For this review, take the finished solid that the model builds, in its own axes (mm). Face numbers are marked on the shaded views. Round coordinates to 2 decimals unless told otherwise and drop trailing zeros. Order: outer loops, then holes, each group sorted by start corner. A loop starts at its lowest first (then second) coordinate and runs counter-clockwise, first axis right, second up. Notation, with made-up numbers: (8, 83) - (35, 83) arc R30 ccw to (35, 108) - close; hole circle Ø1 at (54, 15.25). An arc over 180 degrees is marked (long way). Write each question's results on one line, items separated by ' | '. Start each with the question number.
(1) Take a section at A-A, the plane y = -29. Give the boundary of the cut face in (x, z), plus the area to 3 significant figures.
(2) Take a section at C-C, the plane y = -7.5. Give the boundary of the cut face in (x, z).
(3) For L1, parallel to Y at x = 146, z = 10.25; L2, parallel to Y at x = 156.5, z = 12.55; L3, parallel to Y at x = 128, z = 2.5, list the stretches that pass through material, from the lowest coordinate up. Write a range as from..to.
(4) Take a section at B-B, the plane x = 118. Give the boundary of the cut face in (y, z), plus the area to 3 significant figures.
(5) Insertion check: pin 1 Ø1.2 at (y, z) = (29, 1.5) entering from -X; pin 2 Ø13.5 at (x, y) = (-15.5, -15.5) entering from +Z; pin 3 Ø2.5 at (y, z) = (1, 10.5) entering from +X; pin 4 Ø3 at (x, y) = (156.5, 29) entering from +Z. Each pin has a flat end and moves straight along its axis. Give the tip position at first contact, or say it passes through.
(6) Take a section at D-D, the plane x = -5. Give the boundary of the cut face in (y, z).
(7) Draft analysis for pull direction Z (two halves, no side actions). For the marked faces 1, 2, 3 and 4, state which applies: pulls with the +Z half, pulls with the -Z half, needs draft (parallel to the pull), parting line crosses it, or undercut.
```python
from build123d import *

# Parameters (mm, degrees)
CROQUIS1_W                        = 103
CROQUIS1_H                        = 103
CROQUIS1_R                        = 2.5
SALIENTE_EXTRUIR1_DEPTH           = 15
REDONDEO2_R                       = 51.5
CROQUIS2_W                        = 15
CROQUIS2_H                        = 103
SALIENTE_EXTRUIR2_DEPTH           = 120
CROQUIS3_R                        = 4.25
CORTAR_EXTRUIR1_DEPTH             = 8
SALIENTE_EXTRUIR3_START           = -223
SALIENTE_EXTRUIR3_DEPTH           = 223
CORTAR_EXTRUIR2_DEPTH             = 181.53669987
CORTAR_EXTRUIR2_DEPTH_BACK        = 181.53669987
REDONDEO3_START                   = -23.965772234
REDONDEO3_DEPTH                   = 195.465772234
REDONDEO3_START_2                 = -45.024993159
REDONDEO3_2_DEPTH                 = 21.059220925
REDONDEO3_START_3                 = 15
REDONDEO3_3_DEPTH                 = 9
REDONDEO4_R                       = 10
CORTAR_EXTRUIR3_REACH             = 182.537
CROQUIS6_R                        = 4.25
CORTAR_EXTRUIR3_DIRECTION_2_DEPTH = 181.536699978
CORTAR_EXTRUIR4_DEPTH             = 231.022281636
CORTAR_EXTRUIR4_DEPTH_BACK        = 40
CROQUIS7_W                        = 5
CROQUIS7_H                        = 80
CROQUIS10_R                       = 4.25
CORTAR_EXTRUIR5_DEPTH             = 10
CROQUIS11_R                       = 2.5
CORTAR_EXTRUIR6_DEPTH             = 180.536904387
CROQUIS12_W                       = 16
CROQUIS12_H                       = 24
CROQUIS12_W_2                     = 12
CROQUIS12_H_2                     = 20
SALIENTE_EXTRUIR4_DEPTH           = 171.5
CORTAR_EXTRUIR7_DEPTH             = 4
CROQUIS14_W                       = 242.583484446
CROQUIS14_H                       = 103.867159029
CORTAR_EXTRUIR8_DEPTH             = 8


with BuildPart() as part:
    # Croquis1 → Saliente-Extruir1 (new body)
    with BuildSketch(Plane.XY):
        Rectangle(CROQUIS1_W, CROQUIS1_H)
        with Locations((15.5, 15.5)):
            Circle(CROQUIS1_R, mode=Mode.SUBTRACT)
        with Locations((-15.5, 15.5)):
            Circle(CROQUIS1_R, mode=Mode.SUBTRACT)
        with Locations((-15.5, -15.5)):
            Circle(CROQUIS1_R, mode=Mode.SUBTRACT)
        with Locations((15.5, -15.5)):
            Circle(CROQUIS1_R, mode=Mode.SUBTRACT)
    extrude(amount=SALIENTE_EXTRUIR1_DEPTH)

    # Redondeo2
    redondeo2_edges = [part.edges().sort_by_distance(p)[0] for p in [
        (-51.5, -51.5, 7.5),
        (-51.5, 51.5, 7.5),
    ]]
    fillet(redondeo2_edges, radius=REDONDEO2_R - 0.0001)  # a hair under: the kernel refuses the full size

    # Croquis2 → Saliente-Extruir2 (add)
    with BuildSketch(Plane(origin=(51.5, 0, 0), x_dir=(0, 0, -1), z_dir=(1, 0, 0))):
        with Locations((-7.5, 0)):
            Rectangle(CROQUIS2_W, CROQUIS2_H)
    extrude(amount=SALIENTE_EXTRUIR2_DEPTH)

    # Croquis3 → Cortar-Extruir1 (cut)
    with BuildSketch(Plane.XY.offset(15)):
        with Locations((-15.5, 15.5)):
            Circle(CROQUIS3_R)
        with Locations((15.5, 15.5)):
            Circle(CROQUIS3_R)
        with Locations((15.5, -15.5)):
            Circle(CROQUIS3_R)
        with Locations((-15.5, -15.5)):
            Circle(CROQUIS3_R)
    extrude(amount=-CORTAR_EXTRUIR1_DEPTH, mode=Mode.SUBTRACT)

    # Croquis4 → Saliente-Extruir3 (add)
    with BuildSketch(Plane(origin=(171.5, 0, 0), x_dir=(0, 0, -1), z_dir=(1, 0, 0)).offset(SALIENTE_EXTRUIR3_START)):
        Polygon((-15, -19), (-15, -25), (-23, -25), (-23, 25), (-15, 25), (-15, 19), (-19, 19), (-19, -19), align=None)
    extrude(amount=SALIENTE_EXTRUIR3_DEPTH)

    # Croquis5 → Cortar-Extruir2 (cut, two sides: drawn at the far end of the back side and taken through both)
    with BuildSketch(Plane(origin=(0, 0, 0), x_dir=(-1, 0, 0), z_dir=(0, 0, -1)).offset(-CORTAR_EXTRUIR2_DEPTH_BACK)):
        with BuildLine():
            Line((40.930864284, 31.255629077), (61.422564692, 30.315306135))
            Line((61.422564692, 30.315306135), (63.075048064, -35.056936027))
            Line((63.075048064, -35.056936027), (38.432028807, -34.281615507))
            ThreePointArc((38.432028807, -34.281615507), (48.122237498, -18.343943366), (51.5, 0))
            ThreePointArc((51.5, 0), (48.786214808, 16.497128377), (40.930864284, 31.255629077))
        make_face()
    extrude(amount=CORTAR_EXTRUIR2_DEPTH + CORTAR_EXTRUIR2_DEPTH_BACK, mode=Mode.SUBTRACT)

    # Redondeo3: read off the stored shape, not the designer's step
    # Redondeo3 outline → Redondeo3 (add)
    with BuildSketch(Plane.YZ.offset(REDONDEO3_START)):
        with BuildLine():
            Line((-25, 15), (-25, 23))
            ThreePointArc((-25, 23), (-28.473403651, 17.254033308), (-34.797958971, 15))
            Line((-34.797958971, 15), (-25, 15))
        make_face()
        with BuildLine():
            ThreePointArc((34.797958971, 15), (28.473403651, 17.254033308), (25, 23))
            Line((25, 23), (25, 15))
            Line((25, 15), (34.797958971, 15))
        make_face()
    extrude(amount=REDONDEO3_DEPTH)

    # Redondeo3 2 outline → Redondeo3 2 (add)
    with BuildSketch(Plane.YZ.offset(REDONDEO3_START_2)):
        with BuildLine():
            ThreePointArc((34.797958971, 15), (28.473403651, 17.254033308), (25, 23))
            Line((25, 23), (25, 15))
            Line((25, 15), (34.797958971, 15))
        make_face()
        with BuildLine():
            Line((-25, 15), (-25, 23))
            ThreePointArc((-25, 23), (-28.473403651, 17.254033308), (-34.797958971, 15))
            Line((-34.797958971, 15), (-25, 15))
        make_face()
    extrude(amount=REDONDEO3_2_DEPTH)

    # Redondeo3 3 outline → Redondeo3 3 (cut)
    with BuildSketch(Plane.XY.offset(REDONDEO3_START_3)):
        with BuildLine():
            Line((-45.024993159, -36), (-36.827299657, -36))
            ThreePointArc((-36.827299657, -36), (-41.294060795, -30.774186311), (-45.024993083, -24.999999958))
            Line((-45.024993083, -24.999999958), (-45.024993159, -36))
        make_face()
        with BuildLine():
            Line((-45.024993159, 36), (-45.024993083, 24.999999958))
            ThreePointArc((-45.024993083, 24.999999958), (-41.294060795, 30.774186311), (-36.827299657, 36))
            Line((-36.827299657, 36), (-45.024993159, 36))
        make_face()
    extrude(amount=REDONDEO3_3_DEPTH, mode=Mode.SUBTRACT)

    # Redondeo4
    redondeo4_edges = [part.edges().sort_by_distance(p)[0] for p in [
        (63.237503445, -25, 23),
        (63.237503445, 25, 23),
    ]]
    fillet(redondeo4_edges, radius=REDONDEO4_R)

    # Croquis6 → Cortar-Extruir3 (cut, up to next)
    with BuildSketch(Plane.XY.offset(23), mode=Mode.PRIVATE) as cortar_extruir3_sk1:
        with Locations((15.5, 15.5)):
            Circle(CROQUIS6_R)
    cortar_extruir3_tool1 = extrude(cortar_extruir3_sk1.sketch, amount=-CORTAR_EXTRUIR3_REACH, mode=Mode.PRIVATE) & part.part
    # Croquis6 → Cortar-Extruir3 (cut, up to next)
    with BuildSketch(Plane.XY.offset(23), mode=Mode.PRIVATE) as cortar_extruir3_sk2:
        with Locations((-15.5, 15.5)):
            Circle(CROQUIS6_R)
    cortar_extruir3_tool2 = extrude(cortar_extruir3_sk2.sketch, amount=-CORTAR_EXTRUIR3_REACH, mode=Mode.PRIVATE) & part.part
    # Croquis6 → Cortar-Extruir3 (cut, up to next)
    with BuildSketch(Plane.XY.offset(23), mode=Mode.PRIVATE) as cortar_extruir3_sk3:
        with Locations((15.5, -15.5)):
            Circle(CROQUIS6_R)
    cortar_extruir3_tool3 = extrude(cortar_extruir3_sk3.sketch, amount=-CORTAR_EXTRUIR3_REACH, mode=Mode.PRIVATE) & part.part
    # Croquis6 → Cortar-Extruir3 (cut, up to next)
    with BuildSketch(Plane.XY.offset(23), mode=Mode.PRIVATE) as cortar_extruir3_sk4:
        with Locations((-15.5, -15.5)):
            Circle(CROQUIS6_R)
    cortar_extruir3_tool4 = extrude(cortar_extruir3_sk4.sketch, amount=-CORTAR_EXTRUIR3_REACH, mode=Mode.PRIVATE) & part.part
    add(cortar_extruir3_tool1.solids().sort_by_distance((15.5, 15.5, 23))[0], mode=Mode.SUBTRACT)
    add(cortar_extruir3_tool2.solids().sort_by_distance((-15.5, 15.5, 23))[0], mode=Mode.SUBTRACT)
    add(cortar_extruir3_tool3.solids().sort_by_distance((15.5, -15.5, 23))[0], mode=Mode.SUBTRACT)
    add(cortar_extruir3_tool4.solids().sort_by_distance((-15.5, -15.5, 23))[0], mode=Mode.SUBTRACT)

    # Croquis6 → Cortar-Extruir3 direction 2 (cut)
    with BuildSketch(Plane.XY.offset(23)):
        with Locations((15.5, 15.5)):
            Circle(CROQUIS6_R)
        with Locations((-15.5, 15.5)):
            Circle(CROQUIS6_R)
        with Locations((15.5, -15.5)):
            Circle(CROQUIS6_R)
        with Locations((-15.5, -15.5)):
            Circle(CROQUIS6_R)
    extrude(amount=CORTAR_EXTRUIR3_DIRECTION_2_DEPTH, mode=Mode.SUBTRACT)

    # Croquis7 → Cortar-Extruir4 (cut, two sides: drawn at the far end of the back side and taken through both)
    with BuildSketch(Plane(origin=(171.5, 0, 0), x_dir=(0, 0, -1), z_dir=(1, 0, 0)).offset(-CORTAR_EXTRUIR4_DEPTH_BACK)):
        with Locations((-9.5, 0)):
            Rectangle(CROQUIS7_W, CROQUIS7_H)
    extrude(amount=CORTAR_EXTRUIR4_DEPTH + CORTAR_EXTRUIR4_DEPTH_BACK, mode=Mode.SUBTRACT)

    # Croquis10 → Cortar-Extruir5 (cut)
    with BuildSketch(Plane.XY.offset(23)):
        with Locations((156.5, 29)):
            Circle(CROQUIS10_R)
        with Locations(Location((156.5, -29, 0), (0, 0, 31.206732466))):
            Circle(CROQUIS10_R)
    extrude(amount=-CORTAR_EXTRUIR5_DEPTH, mode=Mode.SUBTRACT)

    # Croquis11 → Cortar-Extruir6 (cut, through all)
    with BuildSketch(Plane.XY.offset(13)):
        with Locations((156.5, 29)):
            Circle(CROQUIS11_R)
        with Locations((156.5, -29)):
            Circle(CROQUIS11_R)
    extrude(amount=-CORTAR_EXTRUIR6_DEPTH, mode=Mode.SUBTRACT)

    # Croquis12 → Saliente-Extruir4 (add)
    with BuildSketch(Plane(origin=(171.5, 0, 0), x_dir=(0, 0, -1), z_dir=(1, 0, 0))):
        with Locations((-8, -63.5)):
            Rectangle(CROQUIS12_W, CROQUIS12_H)
        with Locations((-8, -63.5)):
            Rectangle(CROQUIS12_W_2, CROQUIS12_H_2, mode=Mode.SUBTRACT)
    extrude(amount=-SALIENTE_EXTRUIR4_DEPTH)

    # Croquis13 → Cortar-Extruir7 (cut)
    with BuildSketch(Plane(origin=(0, 0, 0), x_dir=(-1, 0, 0), z_dir=(0, 0, -1))):
        Polygon((-156.5, 24.381197846), (-152.5, 26.690598923), (-152.5, 31.309401077), (-156.5, 33.618802154), (-160.5, 31.309401077), (-160.5, 26.690598923), align=None)
        Polygon((-152.5, -26.690598923), (-156.5, -24.381197846), (-160.5, -26.690598923), (-160.5, -31.309401077), (-156.5, -33.618802154), (-152.5, -31.309401077), align=None)
    extrude(amount=-CORTAR_EXTRUIR7_DEPTH, mode=Mode.SUBTRACT)

    # Croquis14 → Cortar-Extruir8 (cut)
    with BuildSketch(Plane.XY.offset(23)):
        with Locations((50.208257777, 0.433579514)):
            Rectangle(CROQUIS14_W, CROQUIS14_H)
    extrude(amount=-CORTAR_EXTRUIR8_DEPTH, mode=Mode.SUBTRACT)


solid = part.part
```
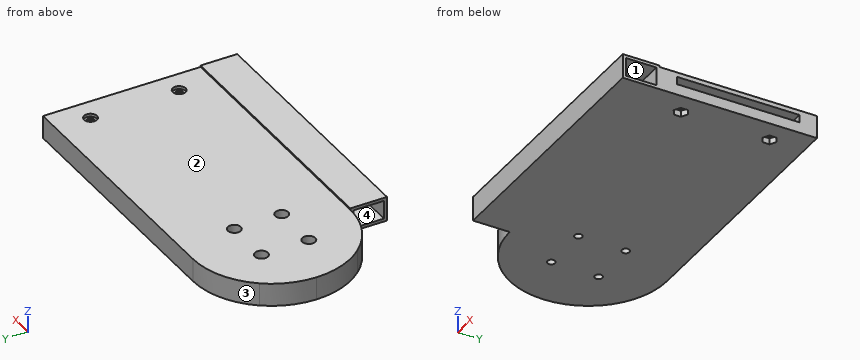
Results below:
1) outline: (-42.56, 0) - (152.5, 0) - (152.5, 4) - (154, 4) - (154, 7) - (131.5, 7) - (131.5, 12) - (154, 12) - (154, 13) - (152.25, 13) - (152.25, 15) - (-42.56, 15) - close; (159, 4) - (160.5, 4) - (160.5, 0) - (171.5, 0) - (171.5, 7) - (159, 7) - close; (159, 12) - (171.5, 12) - (171.5, 15) - (160.75, 15) - (160.75, 13) - (159, 13) - close | area: 2,940 mm^2
2) outline: (-50.95, 0) - (171.5, 0) - (171.5, 7) - (131.5, 7) - (131.5, 12) - (171.5, 12) - (171.5, 15) - (-50.95, 15) - close
3) L1: y = -75.5..-73.5, -53.5..-40, 40..51.5 | L2: y = -75.5..-73.5, -53.5..-31.5, -26.5..26.5, 31.5..51.5 | L3: y = -75.5..-73.5, -53.5..51.5
4) outline: (-75.5, 0) - (51.5, 0) - (51.5, 15) - (-51.5, 15) - (-51.5, 16) - (-75.5, 16) - close; hole (-73.5, 2) - (-53.5, 2) - (-53.5, 14) - (-73.5, 14) - close | area: 1,690 mm^2
5) pin 1: stops at x = -42.96 | pin 2: stops at z = 15 | pin 3: stops at x = 131.5 | pin 4: passes through
6) outline: (-51.26, 0) - (51.26, 0) - (51.26, 15) - (-51.26, 15) - close
7) face 1: undercut | face 2: pulls with the +Z half | face 3: needs draft | face 4: undercut
